```python
from build123d import *

# Parameters (mm, degrees)
ESQUISSE1_R             = 5
BOSS_EXTRU_1_DEPTH      = 5
ESQUISSE2_R             = 3
ENL_V_MAT_EXTRU_1_DEPTH = 3
ESQUISSE9_R             = 1.5
ENL_V_MAT_EXTRU_2_DEPTH = 3
CHANFREIN1_SIZE         = 1


with BuildPart() as part:
    # Esquisse1 → Boss.-Extru.1 (new body)
    with BuildSketch(Plane.XY):
        Circle(ESQUISSE1_R)
    extrude(amount=BOSS_EXTRU_1_DEPTH)

    # Esquisse2 → Enlèv. mat.-Extru.1 (cut)
    with BuildSketch(Plane.XY.offset(5)):
        Circle(ESQUISSE2_R)
    extrude(amount=-ENL_V_MAT_EXTRU_1_DEPTH, mode=Mode.SUBTRACT)

    # Esquisse3 → Enlèvement de matière-Révolution1 (revolve, cut)
    with BuildSketch(Plane(origin=(0, 0, 0), x_dir=(0, 0, -1), z_dir=(1, 0, 0)), mode=Mode.PRIVATE) as enl_vement_de_mati_re_r_volution1_sk:
        with BuildLine():
            Line((0, 5), (-1, 5))
            ThreePointArc((-1, 5), (-0.292893219, 4.707106781), (0, 4))
            Line((0, 4), (0, 5))
        make_face()
        with BuildLine():
            Line((-4, 5), (-5, 5))
            Line((-5, 5), (-5, 4))
            ThreePointArc((-5, 4), (-4.707106781, 4.707106781), (-4, 5))
        make_face()
    revolve(enl_vement_de_mati_re_r_volution1_sk.sketch.rotate(Axis((0, 0, 5), (0, 0, -1)), 90), axis=Axis((0, 0, 5), (0, 0, -1)), mode=Mode.SUBTRACT)

    # Esquisse9 → Enlèv. mat.-Extru.2 (cut)
    with BuildSketch(Plane(origin=(0, 0, 0), x_dir=(-1, 0, 0), z_dir=(0, 0, -1))):
        Circle(ESQUISSE9_R)
    extrude(amount=-ENL_V_MAT_EXTRU_2_DEPTH, mode=Mode.SUBTRACT)

    # Chanfrein1
    chanfrein1_edges = [part.edges().sort_by_distance(p)[0] for p in [
        (1.5, 0, 0),
    ]]
    chamfer(chanfrein1_edges, length=CHANFREIN1_SIZE)


solid = part.part
```
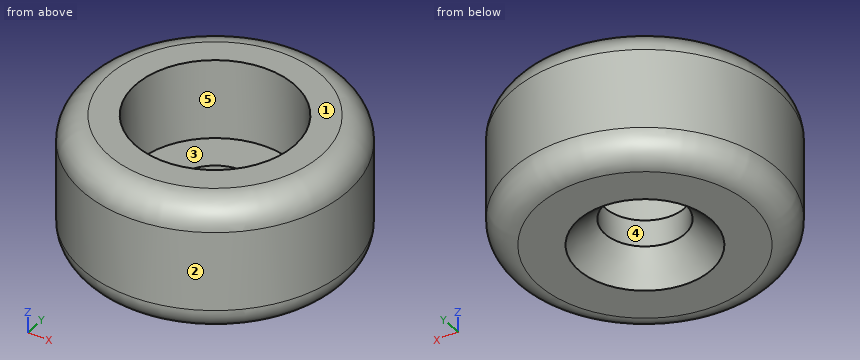
Design review of the part built by this model. Coordinates are the model's own, in mm. Face numbers are marked on the shaded views. A direction names the side the tool comes from. Round coordinates to 2 decimals unless told otherwise and drop trailing zeros. Order: outer loops, then holes, each group sorted by start corner. A loop starts at its lowest first (then second) coordinate and runs counter-clockwise, first axis right, second up. Notation, with made-up numbers: (44.5, 15.25) - (49.5, 15.25) arc R33 ccw to (49.5, 51.25) - close; hole circle Ø10 at (-22, 82.25). An arc over 180 degrees is marked (long way). Return JSON: item names as keys, results as strings.
Q1. Consider section C-C on z = 3.3. Write out the cut boundary in (x, y), plus the area to 3 significant figures.
Computed values:
{"outline": "circle Ø10 at (0, 0); hole circle Ø6 at (0, 0)", "area": "50.3 mm2"}
Q2. Wall thickness on L1, parallel to Y at x = 0, z = 1.8; L2, parallel to Y at x = 0, z = 3.4; L3, parallel to X at y = 1.25, z = 1.8: over which ranges is each line inside the solid? List them lowest first. Write a range as [from, to].
Computed values:
{"L1": "y = [-5, -1.5], [1.5, 5]", "L2": "y = [-5, -3], [3, 5]", "L3": "x = [-4.84, -0.83], [0.83, 4.84]"}
Q3. For pin 1 Ø3.5 at (x, y) = (0, 0) entering from -Z, flat-tipped, find the tip position at first contact; note if it passes through.
Computed values:
{"pin 1": "stops at z = 0.75"}
Q4. Consider section D-D on z = 1.75. Write out the cut boundary in (x, y).
Computed values:
{"outline": "circle Ø10 at (0, 0); hole circle Ø3 at (0, 0)"}
Q5. Consider section A-A on y = 0. Write out the cut boundary in (x, z).
Computed values:
{"outline": "(-5, 1) arc R1 ccw to (-4, 0) - (-2.5, 0) - (-1.5, 1) - (-1.5, 2) - (-3, 2) - (-3, 5) - (-4, 5) arc R1 ccw to (-5, 4) - close; (1.5, 1) - (2.5, 0) - (4, 0) arc R1 ccw to (5, 1) - (5, 4) arc R1 ccw to (4, 5) - (3, 5) - (3, 2) - (1.5, 2) - close"}
Q6. Machinability: for the marked faces 4 and 5, which of the approach directions +Z, -Z, +X, -X, +Y, -Y give a long, thin tool a straight path to every point of the face, cutting with its end or side? Answer none if there is none.
Computed values:
{"face 4": "+Z, -Z", "face 5": "+Z"}
Q7. The part is to be moulded in two halves that separate along Y. For the marked faces 1, 2 and 3, say which applies: pulls with the +Y half, pulls with the -Y half, needs draft (parallel to the pull), parting line crosses it, or undercut.
Computed values:
{"face 1": "needs draft", "face 2": "parting line crosses it", "face 3": "undercut"}
